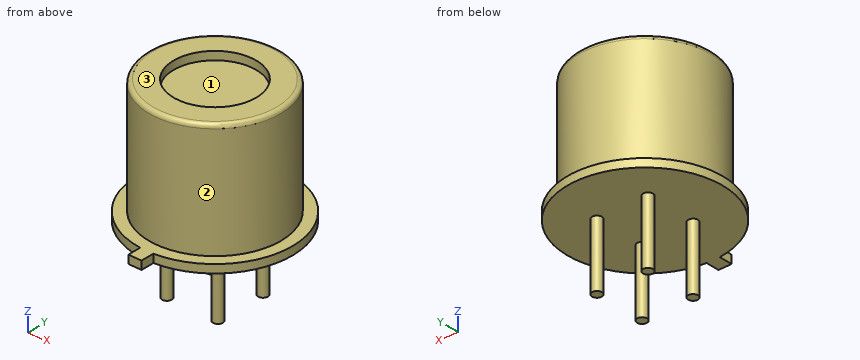
```python
from build123d import *

# Parameters (mm, degrees)
BOSS_EXTRUDE1_DEPTH        = 2
BOSS_EXTRUDE1_DEPTH_BACK   = 2
SKETCH1_R                  = 0.3
BOSS_EXTRUDE1_2_DEPTH      = 2
BOSS_EXTRUDE1_2_DEPTH_BACK = 2
BOSS_EXTRUDE1_3_DEPTH      = 2
BOSS_EXTRUDE1_3_DEPTH_BACK = 2
BOSS_EXTRUDE1_4_DEPTH      = 2
BOSS_EXTRUDE1_4_DEPTH_BACK = 2
BOSS_EXTRUDE2_DEPTH        = 0.5
SKETCH3_R                  = 4
BOSS_EXTRUDE3_DEPTH        = 7
FILLET1_R                  = 0.25
SKETCH4_R                  = 2.5
CUT_EXTRUDE1_DEPTH         = 0.5


with BuildPart() as part:
    # Sketch1 → Boss-Extrude1 (new, two sides: drawn at the far end of the back side and taken through both)
    with BuildSketch(Plane.XY.offset(-BOSS_EXTRUDE1_DEPTH_BACK)):
        with Locations((-1.55, 1.55)):
            Circle(SKETCH1_R)
    extrude(amount=BOSS_EXTRUDE1_DEPTH + BOSS_EXTRUDE1_DEPTH_BACK)



with BuildPart() as body_2:
    # Sketch1 → Boss-Extrude1 2 (new, two sides: drawn at the far end of the back side and taken through both)
    with BuildSketch(Plane.XY.offset(-BOSS_EXTRUDE1_2_DEPTH_BACK)):
        with Locations((-1.55, -1.55)):
            Circle(SKETCH1_R)
    extrude(amount=BOSS_EXTRUDE1_2_DEPTH + BOSS_EXTRUDE1_2_DEPTH_BACK)


with BuildPart() as body_3:
    # Sketch1 → Boss-Extrude1 3 (new, two sides: drawn at the far end of the back side and taken through both)
    with BuildSketch(Plane.XY.offset(-BOSS_EXTRUDE1_3_DEPTH_BACK)):
        with Locations((1.55, 1.55)):
            Circle(SKETCH1_R)
    extrude(amount=BOSS_EXTRUDE1_3_DEPTH + BOSS_EXTRUDE1_3_DEPTH_BACK)


with BuildPart() as body_4:
    # Sketch1 → Boss-Extrude1 4 (new, two sides: drawn at the far end of the back side and taken through both)
    with BuildSketch(Plane.XY.offset(-BOSS_EXTRUDE1_4_DEPTH_BACK)):
        with Locations((1.55, -1.55)):
            Circle(SKETCH1_R)
    extrude(amount=BOSS_EXTRUDE1_4_DEPTH + BOSS_EXTRUDE1_4_DEPTH_BACK)


with BuildPart() as part_1:
    add(part.part)

    add(body_2.part)  # Boss-Extrude2 merges body 2

    add(body_3.part)  # Boss-Extrude2 merges body 3

    add(body_4.part)  # Boss-Extrude2 merges body 4
    # Sketch2 → Boss-Extrude2 (add)
    with BuildSketch(Plane.XY.offset(2)):
        with BuildLine():
            Line((0, -5.5), (0.4, -5.5))
            Line((0.4, -5.5), (0.4, -4.68294779))
            ThreePointArc((0.4, -4.68294779), (0, 4.7), (-0.4, -4.68294779))
            Line((-0.4, -4.68294779), (-0.4, -5.5))
            Line((-0.4, -5.5), (0, -5.5))
        make_face()
    extrude(amount=BOSS_EXTRUDE2_DEPTH)

    # Sketch3 → Boss-Extrude3 (add)
    with BuildSketch(Plane.XY.offset(2.5)):
        Circle(SKETCH3_R)
    extrude(amount=BOSS_EXTRUDE3_DEPTH)

    # Fillet1
    fillet1_edges = [part_1.edges().sort_by_distance(p)[0] for p in [
        (-4, 0, 9.5),
    ]]
    fillet(fillet1_edges, radius=FILLET1_R)

    # Sketch4 → Cut-Extrude1 (cut)
    with BuildSketch(Plane.XY.offset(9.5)):
        Circle(SKETCH4_R)
    extrude(amount=-CUT_EXTRUDE1_DEPTH, mode=Mode.SUBTRACT)


solid = part_1.part
```
Part model, mm, in its own coordinate system. Face numbers are marked on the shaded views. Give positions to 0.01 mm unless a question says otherwise; leave off trailing zeros. Write each loop counter-clockwise with the first axis right and the second up, starting at its lowest first coordinate (ties: lowest second). Pieces come first, ordered by that corner, then holes. Notation, with made-up numbers: M -25.5,-0.75 L 4.5,-0.75 A22 cw 4.5,17.25 Z; hole C 41,17.25 d7. An arc over 180 degrees is marked long. Use CSV: the item, a comma, the result in double quotes.
Item 1: Slice it at C-C on z = 1.75. Write the cut outline in (x, y).
Taken from the geometry:
outline,"C -1.55,-1.55 d0.6; C -1.55,1.55 d0.6; C 1.55,-1.55 d0.6; C 1.55,1.55 d0.6"
Item 2: Pull direction X, two halves, no side cores. Call the marked faces 1, 2 and 3: +X half, -X half, draft (parallel to the pull), parting line (faces both ways), or undercut.
Taken from the geometry:
face 1,"undercut"
face 2,"parting line"
face 3,"draft"
Item 3: Slice it at A-A on x = 0. Write the cut outline in (y, z), plus the area to 3 significant figures.
Taken from the geometry:
outline,"M -5.5,2 L 4.7,2 L 4.7,2.5 L 4,2.5 L 4,9.25 A0.25 ccw 3.75,9.5 L 2.5,9.5 L 2.5,9 L -2.5,9 L -2.5,9.5 L -3.75,9.5 A0.25 ccw -4,9.25 L -4,2.5 L -5.5,2.5 Z"
area,"58.6 mm²"
Item 4: Pin check, flat tips, straight feed: P1, Ø1, axis at x = -0.5, z = 8, coming from the -Y side; P2, Ø6, axis at y = -4, z = 7.5, coming from the -X side. Stop position of each tip, or through.
Taken from the geometry:
P1,"stops at y = -4"
P2,"stops at x = -3.87"
Item 5: Slice it at B-B on y = 0. Write the cut outline in (x, z), plus the area to 3 significant figures.
Taken from the geometry:
outline,"M -4.7,2 L 4.7,2 L 4.7,2.5 L 4,2.5 L 4,9.25 A0.25 ccw 3.75,9.5 L 2.5,9.5 L 2.5,9 L -2.5,9 L -2.5,9.5 L -3.75,9.5 A0.25 ccw -4,9.25 L -4,2.5 L -4.7,2.5 Z"
area,"58.2 mm²"
Item 6: Drill centre lines: probe 1 along Y at (x, z) = (0, 9.2); probe 2 along Z at (x, y) = (-0.25, 2.75); probe 3 along Z at (x, y) = (-1.75, -1). Where is each one in solid material? Low to high.
Taken from the geometry:
probe 1,"y = -4 to -2.5, 2.5 to 4"
probe 2,"z = 2 to 9.5"
probe 3,"z = 2 to 9"
Item 7: Slice it at D-D on z = 6.75. Write the cut outline in (x, y), plus the area to 3 significant figures.
Taken from the geometry:
outline,"C 0,0 d8"
area,"50.3 mm²"
